Can you work these out from the drawing? Everything is in mm from the part's minimum corner. Give positions to 0.01 mm unless a question says otherwise; leave off trailing zeros. Loops run counter-clockwise (first coordinate to the right, second up) from the corner with the lowest first, then second, coordinate; pieces in that order, holes last.
Q1. If we section it at B-B (z = 9.5): Please give me the cut outline in (x, y).
Q2. Will these pins go through, and if not, where does the flat tip stop? P1, Ø0.8, axis at x = 2, y = 71.5, coming from the +Z side; P2, Ø1.4, axis at x = 0.5, y = 64.5, coming from the -Z side; P3, Ø1, axis at x = 0.5, y = 49.5, coming from the +Z side.
Q3. If we section it at C-C (x = 45): Please give me the cut outline in (y, z).
Q4. I need wall thicknesses on line 1 (X direction, y = 93.5, z = 2); line 2 (X direction, y = 77.5, z = 11.5); line 3 (Y direction, x = 57.5, z = 11.25). Which ranges of each line are inside material? Lowest first, please.
Q5. We'd pull the mould along X, two halves only. Please class the marked faces 1 and 2: +X half, -X half, draft (parallel to the pull), parting line (faces both ways), or undercut.
Q6. If we section it at A-A (y = 91): Please give me the cut outline in (x, z), plus the area to 3 significant figures.
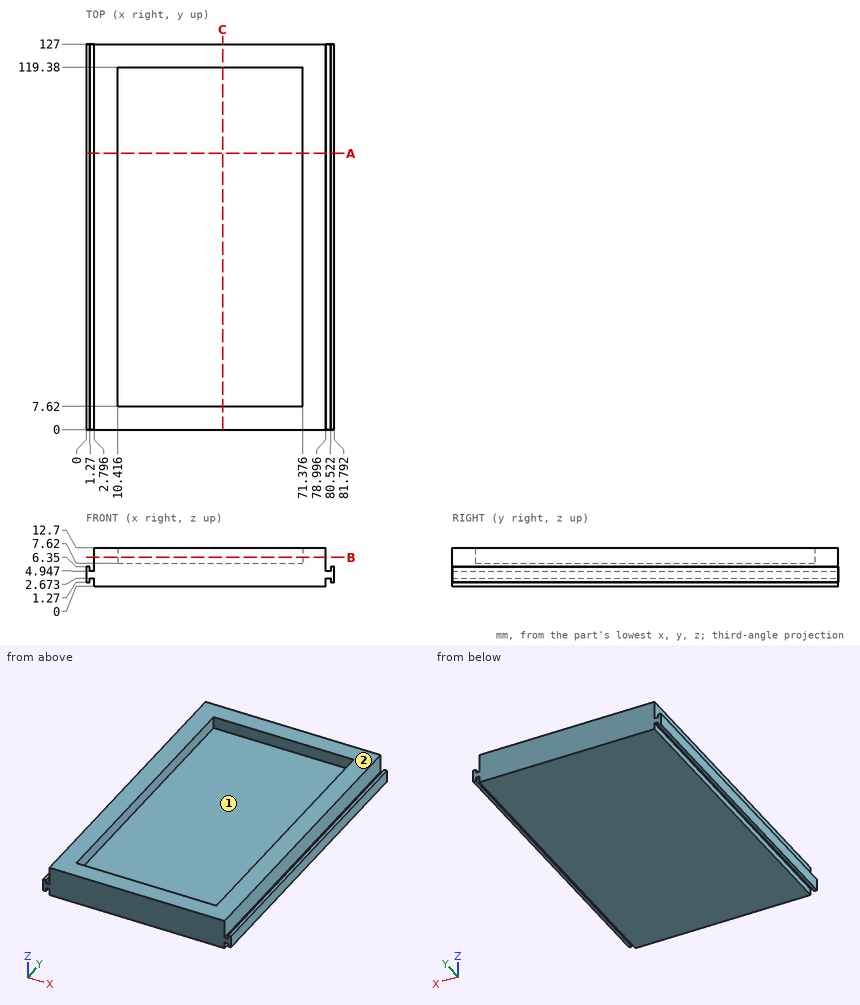
Check sheet entries:
1. outline: (2.8, 0) - (79, 0) - (79, 127) - (2.8, 127) - close; hole (10.42, 7.62) - (71.38, 7.62) - (71.38, 119.38) - (10.42, 119.38) - close
2. P1: stops at z = 4.95
2. P2: stops at z = 1.27
2. P3: stops at z = 6.35
3. outline: (0, 0) - (127, 0) - (127, 12.7) - (119.38, 12.7) - (119.38, 7.62) - (7.62, 7.62) - (7.62, 12.7) - (0, 12.7) - close
4. line 1: x = 0 to 1.27, 2.8 to 79, 80.52 to 81.79
4. line 2: x = 2.8 to 10.42, 71.38 to 79
4. line 3: y = 0 to 7.62, 119.38 to 127
5. face 1: undercut
5. face 2: draft
6. outline: (0, 1.27) - (1.27, 1.27) - (1.27, 2.67) - (2.8, 2.67) - (2.8, 0) - (79, 0) - (79, 2.67) - (80.52, 2.67) - (80.52, 1.27) - (81.79, 1.27) - (81.79, 6.35) - (80.52, 6.35) - (80.52, 4.95) - (79, 4.95) - (79, 12.7) - (71.38, 12.7) - (71.38, 7.62) - (10.42, 7.62) - (10.42, 12.7) - (2.8, 12.7) - (2.8, 4.95) - (1.27, 4.95) - (1.27, 6.35) - (0, 6.35) - close
6. area: 678 mm2
